Work out the finished part from the listing and answer in its coordinate system (mm). Coordinates: 2 decimals unless noted, no trailing zeros. Order: outer loops, then holes, each group sorted by start corner. A loop starts at its lowest first (then second) coordinate and runs counter-clockwise, first axis right, second up. Notation, with made-up numbers: (33, -21) -> (78, -21) arc R31 cw to (78, 3) -> close; hole circle Ø9 at (40.5, -5.75). An arc over 180 degrees is marked (long way). Answer as CSV lines item,"result". Start each with the question number.
Item 1: Each of these flat-tipped pins is pushed along its axis until it touches: pin 1 Ø3 at (x, y) = (45, 0) entering from +Z; pin 2 Ø2 at (x, y) = (43.5, 1) entering from -Z. Where does it stop, or does it pass through?
Item 2: Section B-B (x = 10.5) is taken. Write down the section's boundary in (y, z).
Item 3: Section A-A (z = -2.5) is taken. Write down the section's boundary in (x, y).
Item 4: Straight lines are drawn through the part: L1, parallel to X at y = 1.9, z = -3.5; L2, parallel to X at y = 1.6, z = -3.1; L3, parallel to X at y = 0.4, z = -3. For each, find the intervals that lie inside material, in ascending order.
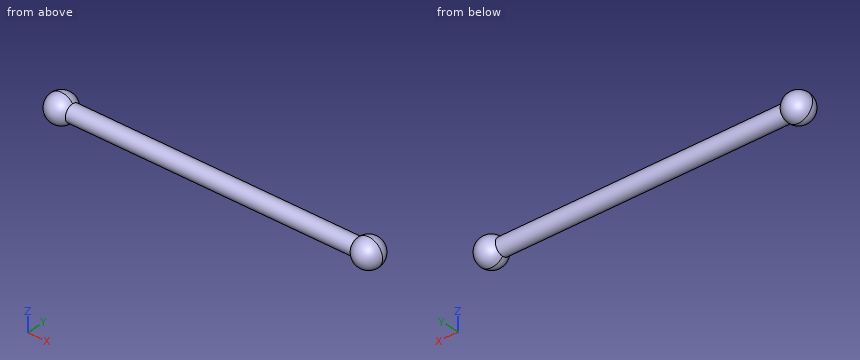
```python
from build123d import *

# Parameters (mm, degrees)
SKETCH5_R   = 1.5
SHAFT_DEPTH = 55


with BuildPart() as part:
    # Sketch4 → Semi-circle Revolve (revolve)
    with BuildSketch(Plane(origin=(0, 0, 0), x_dir=(0, 0, -1), z_dir=(1, 0, 0))):
        with BuildLine():
            Line((0, 0), (2.5, 0))
            Line((2.5, 0), (2.5, -2.5))
            ThreePointArc((2.5, -2.5), (0.732233047, -1.767766953), (0, 0))
        make_face()
    semi_circle_revolve = revolve(axis=Axis((0, 0, -2.5), (0, -1, 0)))

    # Full-circle Mirror: Semi-circle Revolve across plane
    add(semi_circle_revolve.mirror(Plane(origin=(0, 0, 0), x_dir=(0, 0, 1), z_dir=(0, -1, 0))))

    # Sketch5 → Shaft (add)
    with BuildSketch(Plane(origin=(0, 0, 0), x_dir=(0, 0, -1), z_dir=(1, 0, 0))):
        with Locations(Location((2.5, 0, 0), (0, 0, 180))):
            Circle(SKETCH5_R)
    extrude(amount=SHAFT_DEPTH)

    # Sketch6 → Opposite Semi-circle Revolve (revolve)
    with BuildSketch(Plane(origin=(55, 0, 0), x_dir=(0, 0, -1), z_dir=(1, 0, 0))):
        with BuildLine():
            Line((0, 0), (2.5, 0))
            Line((2.5, 0), (2.5, -2.5))
            ThreePointArc((2.5, -2.5), (0.732233047, -1.767766953), (0, 0))
        make_face()
    opposite_semi_circle_revolve = revolve(axis=Axis((55, 0, -2.5), (0, -1, 0)))

    # Opposite Full-circle Mirror: Opposite Semi-circle Revolve across plane
    add(opposite_semi_circle_revolve.mirror(Plane(origin=(55, 0, 0), x_dir=(0, 0, 1), z_dir=(0, 1, 0))))


solid = part.part
```
Checked values:
1,pin 1,"stops at z = -1"
1,pin 2,"stops at z = -4"
2,outline,"circle Ø3 at (0, -2.5)"
3,outline,"(2, -1.5) -> (53, -1.5) arc R2.5 ccw (long way) to (53, 1.5) -> (2, 1.5) arc R2.5 ccw (long way) to start"
4,L1,"x = -1.28 to 1.28, 53.72 to 56.28"
4,L2,"x = -1.82 to 1.82, 53.18 to 56.82"
4,L3,"x = -2.42 to 57.42"
